Answer from the drawing. Dimensions are ordinates in mm from the lowest x, y and z of the part. A direction names the side the tool comes from. Round coordinates to 2 decimals unless told otherwise and drop trailing zeros. Order: outer loops, then holes, each group sorted by start corner. A loop starts at its lowest first (then second) coordinate and runs counter-clockwise, first axis right, second up. Notation, with made-up numbers: M -39.75,39.5 L 8.25,39.5 A9 cw 8.25,50.5 Z; hole C -17,-3 d11. An arc over 180 degrees is marked long. Write item = value, one per line. Start each with the question number.
(1) Straight lines are drawn through the part: probe 1 along Y at (x, z) = (4.75, 0.95); probe 2 along X at (y, z) = (2.75, 0.7); probe 3 along Y at (x, z) = (3, 0.45). For each, find the intervals that lie inside material, in ascending order. Write a range as from..to.
(2) A cutting plane is placed at C-C, the plane z = 0.25. Determine the outline of the cut face in (x, y).
(3) A cutting plane is placed at A-A, the plane x = 8.5. Determine the outline of the cut face in (y, z).
(4) A cutting plane is placed at B-B, the plane y = 2. Determine the outline of the cut face in (x, z), and give its area (3 significant figures).
(5) Which of the six approach directions +Z, -Z, +X, -X, +Y, -Y give full straight-line access (tool end or side, diameter ignored) to the marked faces 4, 5 and 6?
(6) A cutting plane is placed at D-D, the plane y = 4.5. Determine the outline of the cut face in (x, z).
(7) For a pull along X with two mould halves and no side action, classify the marked faces 1, 2 and 3 as released by +X, released by -X, zero draft, split by the parting line, or undercut.
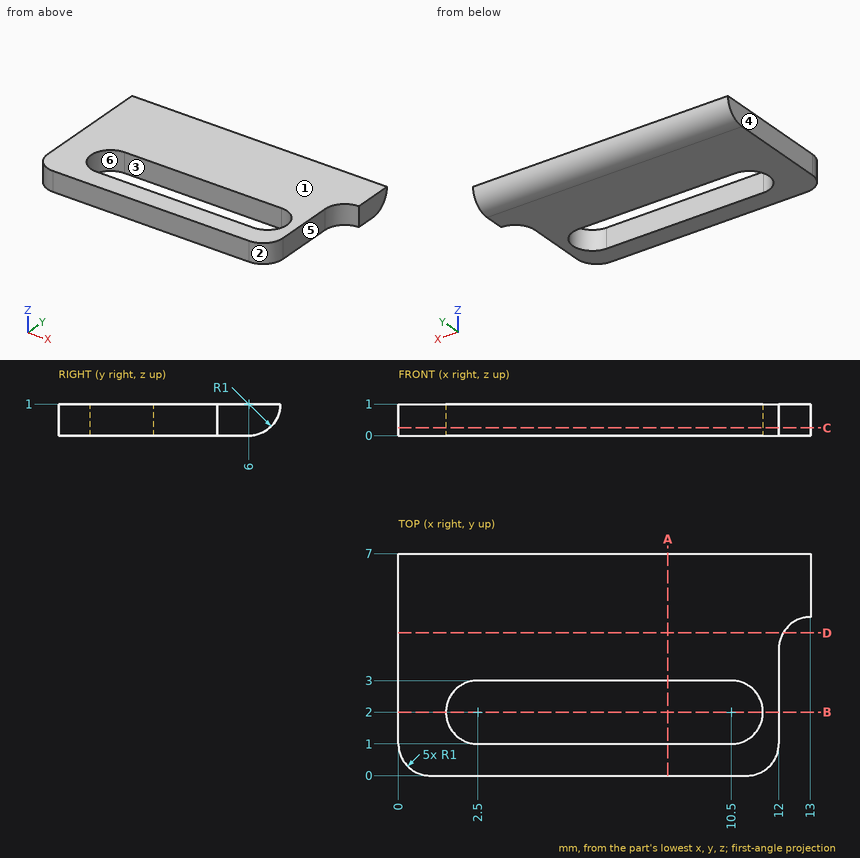
Reported:
q1.probe_1 = 0..1, 3..7
q1.probe_2 = 0..1.84, 11.16..12
q1.probe_3 = 0..1, 3..6.84
q2.outline = M 0,1 A1 ccw 1,0 L 11,0 A1 ccw 12,1 L 12,4 A1 cw 13,5 L 13,6.66 L 0,6.66 Z; hole M 2.5,1 L 10.5,1 A1 ccw 10.5,3 L 2.5,3 A1 ccw Z
q3.outline = M 0,0 L 1,0 L 1,1 L 0,1 Z; M 3,0 L 6,0 A1 ccw 7,1 L 3,1 Z
q4.outline = M 0,0 L 1.5,0 L 1.5,1 L 0,1 Z; M 11.5,0 L 12,0 L 12,1 L 11.5,1 Z
q4.area = 2.00 mm²
q5.face_4 = +Z, -Z, -X, +Y, -Y
q5.face_5 = +Z, -Z, +X, -Y
q5.face_6 = +Z, -Z
q6.outline = M 0,0 L 12.13,0 L 12.13,1 L 0,1 Z
q7.face_1 = zero draft
q7.face_2 = released by +X
q7.face_3 = undercut
